For this review, take the finished solid that the model builds, in its own axes (mm). Face numbers are marked on the shaded views. A direction names the side the tool comes from. Coordinates: 2 decimals unless noted, no trailing zeros. Write each loop counter-clockwise with the first axis right and the second up, starting at its lowest first coordinate (ties: lowest second). Pieces come first, ordered by that corner, then holes.
1) We need section D-D on y = -19. Write out the cut boundary in (x, z), then the cut area to 3 significant figures.
2) Insertion check: P1, Ø12, axis at x = -2, y = -25, coming from the -Z side; P2, Ø1, axis at y = -64.5, z = 17.5, coming from the +X side; P3, Ø8, axis at x = 20.5, y = -43, coming from the -Z side; P4, Ø5, axis at x = 26.5, y = -46, coming from the +Z side. Each pin has a flat end and moves straight along its axis. Give the tip position at first contact, or say it passes through.
3) For the marked faces 1, 2 and 3, list the 3-axis set-ups (+Z, -Z, +X, -X, +Y, -Y) from which the entire face can be reached by the end or side of a thin tool; tool diameter is ignored.
4) We need section C-C on x = 30. Write out the cut boundary in (y, z), then the cut area to 3 significant figures.
5) We need section A-A on z = 0. Write out the cut boundary in (x, y).
6) We need section B-B on y = -30. Write out the cut boundary in (x, z).
7) To check wall thickness, follow line 1 along Z through (x, y) = (25, -32); line 2 along X through (y, z) = (-33, -20); line 3 along X through (y, z) = (-15, 15). State the ranges of each line that lie inside material, in increasing order.
from build123d import *

# Parameters (mm, degrees)
F0_R     = 23.601402
F1_DEPTH = 76.2
F2_R     = 6.959229
F3_DEPTH = 76.2
F4_R     = 6.59301
F5_DEPTH = 76.2


with BuildPart() as f1:
    # F0 (on Front) → F1 (new body)
    with BuildSketch(Plane.XZ):
        Circle(F0_R)
    extrude(amount=F1_DEPTH)

    # F2 (on Right) → F3 (join)
    with BuildSketch(Plane.YZ):
        with Locations((-34.191292, 0)):
            Circle(F2_R)
    extrude(amount=F3_DEPTH)

    # F4 (on Right) → F5 (join)
    with BuildSketch(Plane.YZ):
        with Locations((-34.327276, 0)):
            Circle(F4_R)
    extrude(amount=-F5_DEPTH)


solid = f1.part
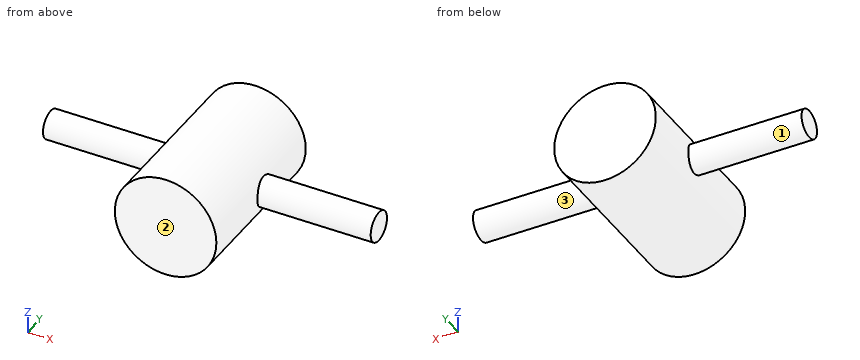
Result:
1. outline: circle Ø47.2 at (0, 0)
1. area: 1,750 mm2
2. P1: stops at z = -23.6
2. P2: stops at x = 16.37
2. P3: stops at z = -16.88
2. P4: passes through
3. face 1: -X
3. face 2: +Z, -Z, +X, -X, -Y
3. face 3: +X
4. outline: circle Ø13.92 at (-34.19, 0)
4. area: 152 mm2
5. outline: (-76.2, -40.92) - (-23.6, -40.92) - (-23.6, -76.2) - (23.6, -76.2) - (23.6, -41.15) - (76.2, -41.15) - (76.2, -27.23) - (23.6, -27.23) - (23.6, 0) - (-23.6, 0) - (-23.6, -27.73) - (-76.2, -27.73) - close
6. outline: (-76.2, -4.97) - (-23.07, -4.97) arc R23.6 ccw to (22.94, -5.56) - (76.2, -5.56) - (76.2, 5.56) - (22.94, 5.56) arc R23.6 ccw to (-23.07, 4.97) - (-76.2, 4.97) - close
7. line 1: z = -6.61 to 6.61
7. line 2: x = -12.53 to 12.53
7. line 3: x = -18.22 to 18.22
